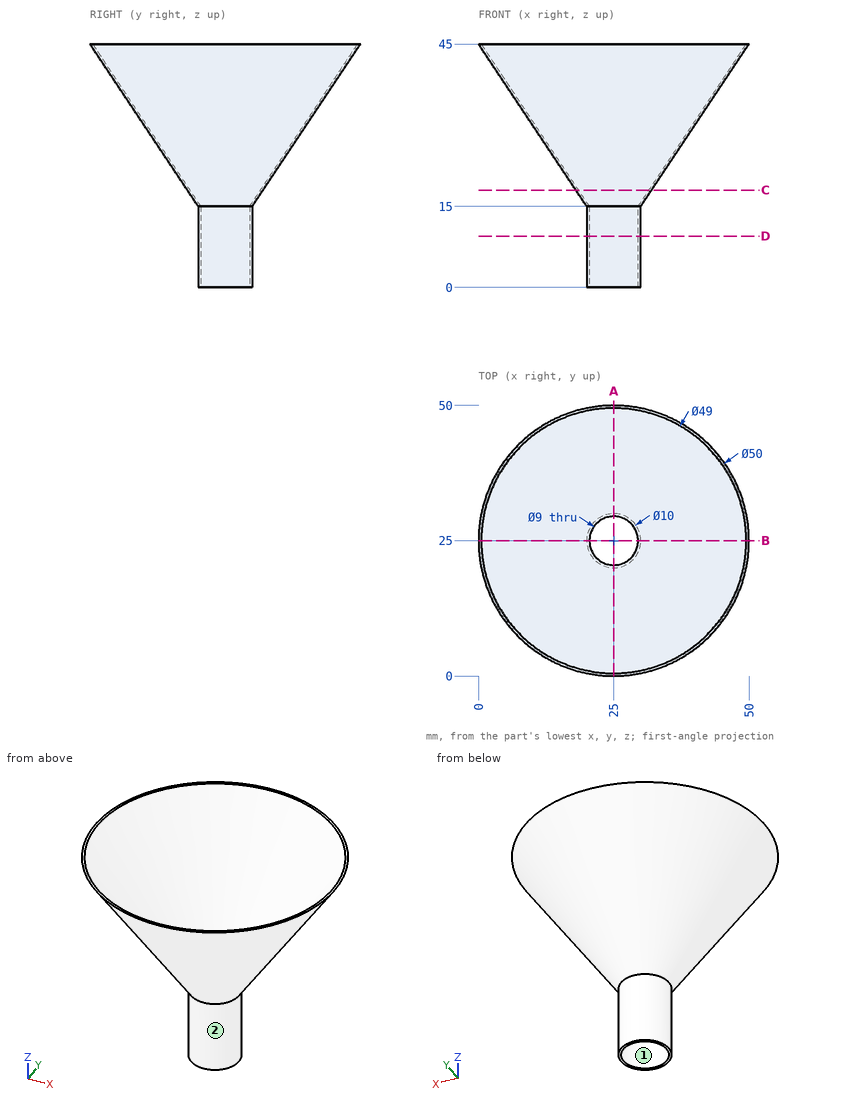
Design review of the part shown in the three views and the two pictorial views. Dimensions are in mm from the part's minimum x, y and z. Round coordinates to 2 decimals unless told otherwise and drop trailing zeros. Loops run counter-clockwise (first coordinate to the right, second up) from the corner with the lowest first, then second, coordinate; pieces in that order, holes last. Notation, with made-up numbers: (75.25, -7) -> (121.25, -7) arc R13 ccw to (121.25, 18) -> close; hole circle Ø6 at (46, 71). An arc over 180 degrees is marked (long way). Answer as CSV lines item,"result".
1) Add section D-D on z = 9.5. Write out the cut boundary in (x, y).
Geometry results:
outline,"circle Ø10 at (25, 25); hole circle Ø9 at (25, 25)"
2) For P1, Ø10, axis at y = 26, z = 13, coming from the -X side; P2, Ø3, axis at x = 26.5, y = 20, coming from the +Z side; P3, Ø1, axis at x = 8.5, y = 26.5, coming from the -Z side; P4, Ø10, axis at y = 8, z = 16.5, coming from the -X side, all flat-tipped, find the tip position at first contact; note any pin that passes through.
Geometry results:
P1,"stops at x = 18.03"
P2,"stops at z = 18.33"
P3,"stops at z = 31.6"
P4,"passes through"
3) Add section A-A on x = 25. Write out the cut boundary in (y, z), plus the area to 3 significant figures.
Geometry results:
outline,"(0, 45) -> (20, 15) -> (20, 0) -> (20.5, 0) -> (20.5, 15) -> (0.5, 45) -> close; (29.5, 0) -> (30, 0) -> (30, 15) -> (50, 45) -> (49.5, 45) -> (29.5, 15) -> close"
area,"45.0 mm²"
4) Draft analysis for pull direction X (two halves, no side actions). For the marked faces 1 and 2, state which applies: pulls with the +X half, pulls with the -X half, needs draft (parallel to the pull), parting line crosses it, or undercut.
Geometry results:
face 1,"undercut"
face 2,"parting line crosses it"
5) To check wall thickness, follow line 1 along Y through (x, z) = (25, 9); line 2 along X through (y, z) = (24, 41); line 3 along Y through (x, z) = (39, 31). State the ranges of each line that lie inside material, in increasing order. Write a range as from..to.
Geometry results:
line 1,"y = 20..20.5, 29.5..30"
line 2,"x = 2.69..3.19, 46.81..47.31"
line 3,"y = 17.97..19.17, 30.83..32.03"
6) Add section C-C on z = 18. Write out the cut boundary in (x, y), plus the area to 3 significant figures.
Geometry results:
outline,"circle Ø14 at (25, 25); hole circle Ø13 at (25, 25)"
area,"21.2 mm²"
